Work out the finished part from the listing and answer in its coordinate system (mm). Face numbers are marked on the shaded views. A direction names the side the tool comes from. Round coordinates to 2 decimals unless told otherwise and drop trailing zeros. Write each loop counter-clockwise with the first axis right and the second up, starting at its lowest first coordinate (ties: lowest second). Pieces come first, ordered by that corner, then holes. Notation, with made-up numbers: M 6.25,-15 L 22.25,-15 A5 cw 22.25,-11 Z; hole C -15,-23.5 d3. An arc over 180 degrees is marked long. One line per item, written item: value. Start each with the question number.
Q1. Find section B-B (z = 25). Write down the section's boundary in (x, y) (3 decimals).
Q2. Given pin 1 Ø3 at (x, y) = (20.5, -9) entering from -Z; pin 2 Ø4 at (y, z) = (-32.5, -7.5) entering from -X; pin 3 Ø2.5 at (x, z) = (34.925, -34.925) entering from +Y; pin 4 Ø5 at (x, y) = (5, -31) entering from +Z, each flat-ended and moving along its own axis, determine where each tip first touches the part or whether it passes through.
Q3. Find section C-C (y = -13.5). Write down the section's boundary in (x, z), and give its area (3 significant figures).
Q4. A tool of negligible diameter and unlimited length cuts with its end or side. For the marked faces 1 and 2, from which of +Z, -Z, +X, -X, +Y, -Y can it reach the whole face along a straight path? Write none if from no direction.
Q5. Consider probe 1 along Y at (x, z) = (33, 30.5); probe 2 along Z at (x, y) = (-5.5, -24); probe 3 along X at (y, z) = (-21.5, -22.5). Determine where each line is inside the solid, lowest interval first.
Q6. The mould has two halves that part along Y. Classify the marked faces 3, 4 and 5: released by +Y, released by -Y, zero draft, split by the parting line, or undercut.
Q7. Find section A-A (x = 0). Write down the section's boundary in (y, z) (3 decimals).
from build123d import *

# Parameters (mm, degrees)
F0_W     = 80.01
F0_H     = 80.01
F0_R     = 2.0447
F1_DEPTH = 3.048
F0_R_2   = 36.83
F2_DEPTH = 35.56
F3_W     = 80.01
F3_H     = 80.01
F3_R     = 2.0447
F3_R_2   = 36.83
F4_DEPTH = 3.048


with BuildPart() as f1:
    # F0 (on Front) → F1 (new body)
    with BuildSketch(Plane.XZ):
        Rectangle(F0_W, F0_H)
        with BuildLine():
            Line((11.355675013, 38.227), (24.6347928475, 38.227))
            Line((24.6347928475, 38.227), (38.227, 38.227))
            Line((38.227, 38.227), (38.227, 24.6347928475))
            Line((38.227, 24.6347928475), (38.227, 11.355675013))
            ThreePointArc((38.227, 11.355675013), (39.463091554, 5.737533355), (39.878, 0))
            ThreePointArc((39.878, 0), (39.463091554, -5.737533355), (38.227, -11.355675013))
            Line((38.227, -11.355675013), (38.227, -24.6347928475))
            Line((38.227, -24.6347928475), (38.227, -38.227))
            Line((38.227, -38.227), (24.6347928475, -38.227))
            Line((24.6347928475, -38.227), (11.355675013, -38.227))
            ThreePointArc((11.355675013, -38.227), (0, -39.878), (-11.355675013, -38.227))
            Line((-11.355675013, -38.227), (-24.6347928475, -38.227))
            Line((-24.6347928475, -38.227), (-38.227, -38.227))
            Line((-38.227, -38.227), (-38.227, -24.6347928475))
            Line((-38.227, -24.6347928475), (-38.227, -11.355675013))
            ThreePointArc((-38.227, -11.355675013), (-39.878, 0), (-38.227, 11.355675013))
            Line((-38.227, 11.355675013), (-38.227, 24.6347928475))
            Line((-38.227, 24.6347928475), (-38.227, 38.227))
            Line((-38.227, 38.227), (-24.6347928475, 38.227))
            Line((-24.6347928475, 38.227), (-11.355675013, 38.227))
            ThreePointArc((-11.355675013, 38.227), (0, 39.878), (11.355675013, 38.227))
        make_face(mode=Mode.SUBTRACT)
        Polygon((38.227, 38.227), (24.6347928475, 38.227), (38.227, 24.6347928475), align=None)
        with Locations((34.925, 34.925)):
            Circle(F0_R, mode=Mode.SUBTRACT)
        Polygon((38.227, -38.227), (38.227, -24.6347928475), (24.6347928475, -38.227), align=None)
        with Locations((34.925, -34.925)):
            Circle(F0_R, mode=Mode.SUBTRACT)
        Polygon((-24.6347928475, -38.227), (-38.227, -24.6347928475), (-38.227, -38.227), align=None)
        with Locations((-34.925, -34.925)):
            Circle(F0_R, mode=Mode.SUBTRACT)
        Polygon((-38.227, 24.6347928475), (-24.6347928475, 38.227), (-38.227, 38.227), align=None)
        with Locations((-34.925, 34.925)):
            Circle(F0_R, mode=Mode.SUBTRACT)
        with BuildLine():
            Line((-11.355675013, 38.227), (11.355675013, 38.227))
            ThreePointArc((11.355675013, 38.227), (0, 39.878), (-11.355675013, 38.227))
        make_face()
        with BuildLine():
            ThreePointArc((39.878, 0), (39.463091554, 5.737533355), (38.227, 11.355675013))
            Line((38.227, 11.355675013), (38.227, -11.355675013))
            ThreePointArc((38.227, -11.355675013), (39.463091554, -5.737533355), (39.878, 0))
        make_face()
        with BuildLine():
            ThreePointArc((-11.355675013, -38.227), (0, -39.878), (11.355675013, -38.227))
            Line((11.355675013, -38.227), (-11.355675013, -38.227))
        make_face()
        with BuildLine():
            Line((-38.227, -11.355675013), (-38.227, 11.355675013))
            ThreePointArc((-38.227, 11.355675013), (-39.878, 0), (-38.227, -11.355675013))
        make_face()
        with BuildLine():
            ThreePointArc((-11.355675013, -38.227), (-28.1980042202, -28.1980042202), (-38.227, -11.355675013))
            Line((-38.227, -11.355675013), (-38.227, -24.6347928475))
            Line((-38.227, -24.6347928475), (-24.6347928475, -38.227))
            Line((-24.6347928475, -38.227), (-11.355675013, -38.227))
        make_face()
        with BuildLine():
            ThreePointArc((-38.227, 11.355675013), (-28.1980042202, 28.1980042202), (-11.355675013, 38.227))
            Line((-11.355675013, 38.227), (-24.6347928475, 38.227))
            Line((-24.6347928475, 38.227), (-38.227, 24.6347928475))
            Line((-38.227, 24.6347928475), (-38.227, 11.355675013))
        make_face()
        with BuildLine():
            Line((38.227, 24.6347928475), (24.6347928475, 38.227))
            Line((24.6347928475, 38.227), (11.355675013, 38.227))
            ThreePointArc((11.355675013, 38.227), (28.1980042202, 28.1980042202), (38.227, 11.355675013))
            Line((38.227, 11.355675013), (38.227, 24.6347928475))
        make_face()
        with BuildLine():
            Line((38.227, -24.6347928475), (38.227, -11.355675013))
            ThreePointArc((38.227, -11.355675013), (28.1980042202, -28.1980042202), (11.355675013, -38.227))
            Line((11.355675013, -38.227), (24.6347928475, -38.227))
            Line((24.6347928475, -38.227), (38.227, -24.6347928475))
        make_face()
    extrude(amount=F1_DEPTH)

    # F0 (on Front) → F2 (join)
    with BuildSketch(Plane.XZ):
        with BuildLine():
            ThreePointArc((38.227, 11.355675013), (28.1980042202, 28.1980042202), (11.355675013, 38.227))
            Line((11.355675013, 38.227), (-11.355675013, 38.227))
            ThreePointArc((-11.355675013, 38.227), (-28.1980042202, 28.1980042202), (-38.227, 11.355675013))
            Line((-38.227, 11.355675013), (-38.227, -11.355675013))
            ThreePointArc((-38.227, -11.355675013), (-28.1980042202, -28.1980042202), (-11.355675013, -38.227))
            Line((-11.355675013, -38.227), (11.355675013, -38.227))
            ThreePointArc((11.355675013, -38.227), (28.1980042202, -28.1980042202), (38.227, -11.355675013))
            Line((38.227, -11.355675013), (38.227, 11.355675013))
        make_face()
        Circle(F0_R_2, mode=Mode.SUBTRACT)
        with BuildLine():
            ThreePointArc((39.878, 0), (39.463091554, 5.737533355), (38.227, 11.355675013))
            Line((38.227, 11.355675013), (38.227, -11.355675013))
            ThreePointArc((38.227, -11.355675013), (39.463091554, -5.737533355), (39.878, 0))
        make_face()
        with BuildLine():
            Line((-38.227, -11.355675013), (-38.227, 11.355675013))
            ThreePointArc((-38.227, 11.355675013), (-39.878, 0), (-38.227, -11.355675013))
        make_face()
        with BuildLine():
            ThreePointArc((-11.355675013, -38.227), (0, -39.878), (11.355675013, -38.227))
            Line((11.355675013, -38.227), (-11.355675013, -38.227))
        make_face()
        with BuildLine():
            Line((-11.355675013, 38.227), (11.355675013, 38.227))
            ThreePointArc((11.355675013, 38.227), (0, 39.878), (-11.355675013, 38.227))
        make_face()
    extrude(amount=F2_DEPTH)

    # F3 (on face) → F4 (join)
    with BuildSketch(Plane.XZ.offset(35.56)):
        Rectangle(F3_W, F3_H)
        Polygon((-38.227, -38.227), (-38.227, -24.6347928475), (-38.227, 24.6347928475), (-38.227, 38.227), (-24.6347928475, 38.227), (24.6347928475, 38.227), (38.227, 38.227), (38.227, 24.6347928475), (38.227, -24.6347928475), (38.227, -38.227), (24.6347928475, -38.227), (-24.6347928475, -38.227), align=None, mode=Mode.SUBTRACT)
        Polygon((-24.6347928475, -38.227), (-38.227, -24.6347928475), (-38.227, -38.227), align=None)
        with Locations((-34.925, -34.925)):
            Circle(F3_R, mode=Mode.SUBTRACT)
        Polygon((-38.227, 38.227), (-38.227, 24.6347928475), (-24.6347928475, 38.227), align=None)
        with Locations((-34.925, 34.925)):
            Circle(F3_R, mode=Mode.SUBTRACT)
        Polygon((38.227, 38.227), (24.6347928475, 38.227), (38.227, 24.6347928475), align=None)
        with Locations((34.925, 34.925)):
            Circle(F3_R, mode=Mode.SUBTRACT)
        Polygon((38.227, -24.6347928475), (24.6347928475, -38.227), (38.227, -38.227), align=None)
        with Locations((34.925, -34.925)):
            Circle(F3_R, mode=Mode.SUBTRACT)
        with BuildLine():
            Line((-38.227, 11.355675013), (-38.227, -11.355675013))
            ThreePointArc((-38.227, -11.355675013), (-28.1980042202, -28.1980042202), (-11.355675013, -38.227))
            Line((-11.355675013, -38.227), (11.355675013, -38.227))
            ThreePointArc((11.355675013, -38.227), (28.1980042202, -28.1980042202), (38.227, -11.355675013))
            Line((38.227, -11.355675013), (38.227, 11.355675013))
            ThreePointArc((38.227, 11.355675013), (28.1980042202, 28.1980042202), (11.355675013, 38.227))
            Line((11.355675013, 38.227), (-11.355675013, 38.227))
            ThreePointArc((-11.355675013, 38.227), (-28.1980042202, 28.1980042202), (-38.227, 11.355675013))
        make_face()
        Circle(F3_R_2, mode=Mode.SUBTRACT)
        with BuildLine():
            ThreePointArc((38.227, -11.355675013), (28.1980042202, -28.1980042202), (11.355675013, -38.227))
            Line((11.355675013, -38.227), (24.6347928475, -38.227))
            Line((24.6347928475, -38.227), (38.227, -24.6347928475))
            Line((38.227, -24.6347928475), (38.227, -11.355675013))
        make_face()
        with BuildLine():
            Line((24.6347928475, 38.227), (11.355675013, 38.227))
            ThreePointArc((11.355675013, 38.227), (28.1980042202, 28.1980042202), (38.227, 11.355675013))
            Line((38.227, 11.355675013), (38.227, 24.6347928475))
            Line((38.227, 24.6347928475), (24.6347928475, 38.227))
        make_face()
        with BuildLine():
            Line((-38.227, 24.6347928475), (-38.227, 11.355675013))
            ThreePointArc((-38.227, 11.355675013), (-28.1980042202, 28.1980042202), (-11.355675013, 38.227))
            Line((-11.355675013, 38.227), (-24.6347928475, 38.227))
            Line((-24.6347928475, 38.227), (-38.227, 24.6347928475))
        make_face()
        with BuildLine():
            Line((-38.227, -11.355675013), (-38.227, -24.6347928475))
            Line((-38.227, -24.6347928475), (-24.6347928475, -38.227))
            Line((-24.6347928475, -38.227), (-11.355675013, -38.227))
            ThreePointArc((-11.355675013, -38.227), (-28.1980042202, -28.1980042202), (-38.227, -11.355675013))
        make_face()
    extrude(amount=F4_DEPTH)


solid = f1.part
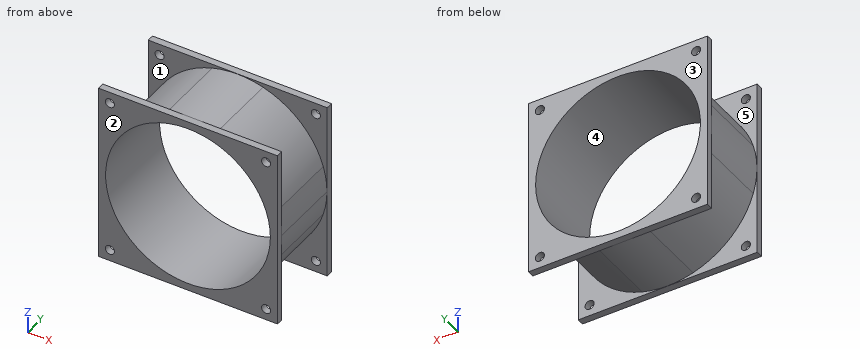
The answers:
1. outline: M -40.005,-38.608 L -27.045,-38.608 L -27.045,0 L -40.005,0 L -40.005,-3.048 L -31.069,-3.048 L -31.069,-35.56 L -40.005,-35.56 Z; M 27.045,-38.608 L 40.005,-38.608 L 40.005,-35.56 L 31.069,-35.56 L 31.069,-3.048 L 40.005,-3.048 L 40.005,0 L 27.045,0 Z
2. pin 1: z = -35.06
2. pin 2: x = -39.5
2. pin 3: through
2. pin 4: z = 39.8
3. outline: C 0,0 d79.76; hole C 0,0 d73.66
3. area: 735 mm2
4. face 1: none
4. face 2: +Z, -Z, +X, -X, -Y
5. probe 1: -38.61 to -35.56, -3.05 to 0
5. probe 2: -39.5 to -36.42, 36.42 to 39.5
5. probe 3: -32.92 to -29.16, 29.16 to 32.92
6. face 3: released by +Y
6. face 4: zero draft
6. face 5: undercut
7. outline: M -38.608,-40.005 L -35.56,-40.005 L -35.56,-39.878 L -3.048,-39.878 L -3.048,-40.005 L 0,-40.005 L 0,-36.83 L -38.608,-36.83 Z; M -38.608,36.83 L 0,36.83 L 0,40.005 L -3.048,40.005 L -3.048,39.878 L -35.56,39.878 L -35.56,40.005 L -38.608,40.005 Z
